Verification items for the finished model (mm, model axes). A direction names the side the tool comes from. Give positions to 0.01 mm unless a question says otherwise; leave off trailing zeros. Loops run counter-clockwise (first coordinate to the right, second up) from the corner with the lowest first, then second, coordinate; pieces in that order, holes last. Notation, with made-up numbers: (58, -23) - (76, -23) arc R20 cw to (76, 3) - close; hole circle Ø3 at (5, 1.25). An arc over 180 degrees is marked (long way). One line per item, written item: value. Start each with the question number.
1. Sectioned sample at C-C (y = 0.5). Record the cut outline in (x, z), plus the area to 3 significant figures.
2. Sectioned sample at A-A (y = -6). Record the cut outline in (x, z), plus the area to 3 significant figures.
3. Sectioned sample at B-B (x = 0). Record the cut outline in (y, z).
4. Gauge pin test, flat ends, axial feed: pin 1 (1.9 mm diameter, centred on x = -10.39, y = 6, fed in from +Z) (1 decimal); pin 2 (1 mm diameter, centred on x = 1, z = 0.5, fed in from -Y); pin 3 (10.5 mm diameter, centred on x = 0, y = 0, fed in from +Z). Record the tip position at first contact, or that the pin passes through.
5. Mould release check, pull along X, two halves, no side actions. Record for faces 1 (the cylindrical face through (0.1, -14.5, 1)), 2 (the cylindrical face through (2.48, 4.34, 0.99)), 3 (the cylindrical face through (5, 0, 1)), 4 (the cylindrical face through (-5, 0, 1)): pulls with the +X half, pulls with the -X half, needs draft (parallel to the pull), parting line crosses it, or undercut.
6. Scan lines: L1, parallel to Y at x = 0, z = 1.4; L2, parallel to Y at x = -9, z = 0.25; L3, parallel to X at y = -8, z = 0.8. Record each from-to range of solid material in increasing order. Write a range as [from, to].
7. Access from +Z, -Z, +X, -X, +Y, -Y to the whole of each face (thin tool, end or side, straight path). Record for faces 5 (the flat face through (-6.04, -4.065, 0.986)), 6 (the flat face through (6.54, -3.2, 0.99)), 7 (the flat face through (6.04, 4.065, 0.986)).
8. Sectioned sample at D-D (x = 11). Record the cut outline in (y, z), plus the area to 3 significant figures.
from build123d import *

# Parameters (mm, degrees)
SKETCH_1_R      = 1.6
SKETCH_1_R_2    = 4
EXTRUDE_1_DEPTH = 2
FILLET_1_R      = 0.5


with BuildPart() as part:
    # ｽｹｯﾁ1 → ﾎﾞｽ - 押し出し1 (new body)
    with BuildSketch(Plane.XY):
        with BuildLine():
            Line((4.058421985, 2.920481295), (8.020984502, 5.208267831))
            ThreePointArc((8.020984502, 5.208267831), (12.557368355, 7.25), (8.520984502, 4.342242427))
            Line((8.520984502, 4.342242427), (4.558421985, 2.054455891))
            ThreePointArc((4.558421985, 2.054455891), (5, 0), (4.558421985, -2.054455891))
            Line((4.558421985, -2.054455891), (8.520984502, -4.342242427))
            ThreePointArc((8.520984502, -4.342242427), (12.557368355, -7.25), (8.020984502, -5.208267831))
            Line((8.020984502, -5.208267831), (4.058421985, -2.920481295))
            ThreePointArc((4.058421985, -2.920481295), (2.5, -4.330127019), (0.5, -4.974937186))
            Line((0.5, -4.974937186), (0.5, -9.550510257))
            ThreePointArc((0.5, -9.550510257), (0, -14.5), (-0.5, -9.550510257))
            Line((-0.5, -9.550510257), (-0.5, -4.974937186))
            ThreePointArc((-0.5, -4.974937186), (-2.5, -4.330127019), (-4.058421985, -2.920481295))
            Line((-4.058421985, -2.920481295), (-8.020984502, -5.208267831))
            ThreePointArc((-8.020984502, -5.208267831), (-12.557368355, -7.25), (-8.520984502, -4.342242427))
            Line((-8.520984502, -4.342242427), (-4.558421985, -2.054455891))
            ThreePointArc((-4.558421985, -2.054455891), (-5, 0), (-4.558421985, 2.054455891))
            Line((-4.558421985, 2.054455891), (-8.520984502, 4.342242427))
            ThreePointArc((-8.520984502, 4.342242427), (-12.557368355, 7.25), (-8.020984502, 5.208267831))
            Line((-8.020984502, 5.208267831), (-4.058421985, 2.920481295))
            ThreePointArc((-4.058421985, 2.920481295), (-2.5, 4.330127019), (-0.5, 4.974937186))
            Line((-0.5, 4.974937186), (-0.5, 9.550510257))
            ThreePointArc((-0.5, 9.550510257), (0, 14.5), (0.5, 9.550510257))
            Line((0.5, 9.550510257), (0.5, 4.974937186))
            ThreePointArc((0.5, 4.974937186), (2.5, 4.330127019), (4.058421985, 2.920481295))
        make_face()
        with Locations((0, 12)):
            Circle(SKETCH_1_R, mode=Mode.SUBTRACT)
        with Locations((10.392304845, 6)):
            Circle(SKETCH_1_R, mode=Mode.SUBTRACT)
        with Locations((10.392304845, -6)):
            Circle(SKETCH_1_R, mode=Mode.SUBTRACT)
        with Locations((0, -12)):
            Circle(SKETCH_1_R, mode=Mode.SUBTRACT)
        with Locations((-10.392304845, -6)):
            Circle(SKETCH_1_R, mode=Mode.SUBTRACT)
        with Locations((-10.392304845, 6)):
            Circle(SKETCH_1_R, mode=Mode.SUBTRACT)
        Circle(SKETCH_1_R_2, mode=Mode.SUBTRACT)
    extrude(amount=EXTRUDE_1_DEPTH)

    # ﾌｨﾚｯﾄ1
    fillet_1_edges = [part.edges().sort_by_distance(p)[0] for p in [
        (0.5, 9.550510257, 1),
        (0.5, 4.974937186, 1),
        (4.058421985, 2.920481295, 1),
        (8.020984502, 5.208267831, 1),
        (8.520984502, 4.342242427, 1),
        (4.558421985, 2.054455891, 1),
        (4.558421985, -2.054455891, 1),
        (8.520984502, -4.342242427, 1),
        (8.020984502, -5.208267831, 1),
        (4.058421985, -2.920481295, 1),
        (0.5, -4.974937186, 1),
        (0.5, -9.550510257, 1),
        (-0.5, -9.550510257, 1),
        (-0.5, -4.974937186, 1),
        (-4.058421985, -2.920481295, 1),
        (-8.020984502, -5.208267831, 1),
        (-8.520984502, -4.342242427, 1),
        (-4.558421985, -2.054455891, 1),
        (-4.558421985, 2.054455891, 1),
        (-8.520984502, 4.342242427, 1),
        (-8.020984502, 5.208267831, 1),
        (-4.058421985, 2.920481295, 1),
        (-0.5, 4.974937186, 1),
        (-0.5, 9.550510257, 1),
    ]]
    fillet(fillet_1_edges, radius=FILLET_1_R)


solid = part.part
Results are:
1. outline: (-4.97, 0) - (-3.97, 0) - (-3.97, 2) - (-4.97, 2) - close; (3.97, 0) - (4.97, 0) - (4.97, 2) - (3.97, 2) - close
1. area: 4.03 mm^2
2. outline: (-12.89, 0) - (-11.99, 0) - (-11.99, 2) - (-12.89, 2) - close; (-8.79, 0) - (-7.89, 0) - (-7.89, 2) - (-8.79, 2) - close; (-0.5, 0) - (0.5, 0) - (0.5, 2) - (-0.5, 2) - close; (7.89, 0) - (8.79, 0) - (8.79, 2) - (7.89, 2) - close; (11.99, 0) - (12.89, 0) - (12.89, 2) - (11.99, 2) - close
2. area: 9.20 mm^2
3. outline: (-14.5, 0) - (-13.6, 0) - (-13.6, 2) - (-14.5, 2) - close; (-10.4, 0) - (-4, 0) - (-4, 2) - (-10.4, 2) - close; (4, 0) - (10.4, 0) - (10.4, 2) - (4, 2) - close; (13.6, 0) - (14.5, 0) - (14.5, 2) - (13.6, 2) - close
4. pin 1: passes through
4. pin 2: stops at y = -14.45
4. pin 3: stops at z = 2
5. face 1: parting line crosses it
5. face 2: undercut
5. face 3: pulls with the +X half
5. face 4: pulls with the -X half
6. L1: y = [-14.5, -13.6], [-10.4, -4], [4, 10.4], [13.6, 14.5]
6. L2: y = [-8.08, -6.79], [-5.21, -3.92], [3.92, 5.21], [6.79, 8.08]
6. L3: x = [-11.89, -8.89], [-0.5, 0.5], [8.89, 11.89]
7. face 5: +Z, -Z, -Y
7. face 6: +Z, -Z
7. face 7: +Z, -Z, +Y
8. outline: (-8.43, 0) - (-7.48, 0) - (-7.48, 2) - (-8.43, 2) - close; (-4.52, 0) - (-3.57, 0) - (-3.57, 2) - (-4.52, 2) - close; (3.57, 0) - (4.52, 0) - (4.52, 2) - (3.57, 2) - close; (7.48, 0) - (8.43, 0) - (8.43, 2) - (7.48, 2) - close
8. area: 7.56 mm^2
